Build history of the part. All positions in model axes, mm. A direction names the side the tool comes from. Coordinates: 2 decimals unless noted, no trailing zeros. Loops run counter-clockwise (first coordinate to the right, second up) from the corner with the lowest first, then second, coordinate; pieces in that order, holes last.
(1) Slice it at D-D (x = 38). Give the cut face in (y, z).
(2) Tool access for faces 4 (the face through (7, 13, 5)), 5 (the face through (-12.43, 14.15, 4.46)), 6 (the face through (35, 22, 5)), 7 (the face through (35, 3, 5)): list every direction of +Z, -Z, +X, -X, +Y, -Y with a clear straight run to the whole face (end or side of a thin tool).
(3) Flat gauge pins, fed straight in: P1, Ø3, axis at x = -6, y = 7, coming from the -Z side; P2, Ø4, axis at x = -3, y = 17.5, coming from the +Z side; P3, Ø5, axis at x = -3.5, z = 5, coming from the -Y side; P4, Ø7.5, axis at x = 39.5, z = 7, coming from the +Y side. Where does each tip first touch, or does it go through?
(4) Wall check: L1, parallel to X at y = 11.25, z = 5; L2, parallel to Y at x = 13, z = 6.25; L3, parallel to Z at x = 19, y = 5.25. Give the ranges that are in metal, low to high.
(5) Slice it at C-C (z = 5.75). Give the number of separate pieces and of enclosed holes in the cut face, and give its area (3 significant figures).
(6) Slice it at A-A (x = 19). Give the cut face in (y, z), and give its area (3 significant figures).
(7) Two-plate mould, pull along X, no slides. Class faces 1 (the face through (20.57, 4.563, 0.723)), 2 (the face through (2, 15, 10)), 3 (the face through (-12.4, 19.82, 4.46)): pulls with the +X half, pulls with the -X half, needs draft (parallel to the pull), parting line crosses it, or undercut.
(8) Slice it at B-B (z = 11.5). Give the cut face in (x, y).
Autodesk Inventor part; units mm, degrees
ref_plane "YZ Plane" through (0, 0, 0) normal (1, 0, 0) x (0, 1, 0)
ref_plane "XZ Plane" through (0, 0, 0) normal (0, 1, 0) x (-1, 0, 0)
ref_plane "XY Plane" through (0, 0, 0) normal (0, 0, 1) x (1, 0, 0)
sketch "Sketch1" plane through (0, 0, 0) normal (0, 0, 1) x (1, 0, 0)
  line L0 (0, 0) -> (0, 25)
  line L1 (0, 25) -> (35, 25)
  line L2 (35, 25) -> (35, 18.75)
  line L3 (35, 18.75) -> (44.5, 18.75)
  line L4 (44.5, 18.75) -> (44.5, 6.25)
  line L5 (44.5, 6.25) -> (35, 6.25)
  line L6 (35, 6.25) -> (35, 0)
  line L7 (35, 0) -> (0, 0)
  point P0 (0, 12.5)
  point P1 (44.5, 12.5)
  dimension "d0" = 25
  dimension "d1" = 35
  dimension "d2" = 12.5
  dimension "d3" = 6.25
  dimension "d4" = 9.5
extrude "Extrusion1" add sketch "Sketch1" along normal blind 10
hole "Hole1" at (40.2, 6.25, 5) direction (0, 1, 0) diameter 3 end through all
chamfer "Chamfer1" distance 2.5 angle 45 1 edges at (44.5, 12.5, 0)
hole "Hole2" at (19, 0, 4.51) direction (0, 1, 0) diameter 8.2 end through all
sketch "Sketch2" plane through (0, 0, 10) normal (0, 0, 1) x (1, 0, 0)
  line L0 (0, 25) -> (35, 25)
  line L1 (35, 0) -> (0, 0)
  line L2 (23.1, 25) -> (23.1, 0)
  line L3 (14.9, 25) -> (14.9, 0)
  line L4 (9, 0) -> (29, 0)
  line L5 (29, 0) -> (29, 25)
  line L6 (29, 25) -> (9, 25)
  line L7 (9, 25) -> (9, 0)
  dimension "d28" = 20
  dimension "d29" = 6
extrude "Extrusion2" add sketch "Sketch2" along normal blind 3
chamfer "Chamfer2" distance 3 angle 45 2 edges at (29, 12.5, 13) (9, 12.5, 13)
sketch "Sketch3" plane through (0, 0, 0) normal (-1, 0, 0) x (0, 0, 1)
  line L0 (10, 0) -> (10, 25)
  line L1 (0, 25) -> (10, 25)
  line L2 (10, 25) -> (10, 9)
  line L3 (10, 9) -> (0, 9)
  line L4 (0, 9) -> (0, 25)
  dimension "d35" = 16
extrude "Extrusion3" add sketch "Sketch3" along normal blind 13
hole "Hole3" at (-5.5, 17, 10) direction (0, 0, -1) diameter 4.5 end through all
sketch "Sketch4" plane through (0, 0, 10) normal (0, 0, 1) x (1, 0, 0)
  circle A0 centre (-5.5, 17) radius 2.25
  line L0 (-13, 25) -> (-13, 9)
  line L1 (-5.5, 19.25) -> (-13, 19.25)
  line L2 (-13, 19.25) -> (-13, 14.75)
  line L3 (-13, 14.75) -> (-5.5, 14.75)
  line L4 (-5.5, 14.75) -> (-5.5, 19.25)
extrude "Extrusion4" cut sketch "Sketch4" against normal through all contours L4 A0 | A0 L3 L0 L1 picked at (-6.2445, 17.0904)
fillet "Fillet1" radius 2 4 edges at (-13, 25, 5) (-13, 19.25, 5) (-13, 14.75, 5) (-13, 9, 5)
sketch "Sketch5" plane through (0, 9, 0) normal (0, -1, 0) x (1, 0, 0)
  line L0 (0, 10) -> (-11, 10)
  line L1 (-13, 10) -> (-13, 0)
  line L2 (-13, 10) -> (-11, 10)
  line L3 (-13, 10) -> (-9.4444, 10)
  line L4 (-13, 7.7985) -> (-13, 10)
  line L5 (-13, 7.7985) -> (-9.4444, 10)
  dimension "d52" = 3.5556
  dimension "d53" = 2.2015
extrude "Extrusion5" cut sketch "Sketch5" against normal through all
fillet "Fillet2" radius 6 1 edges at (0, 0, 5)
sketch "Sketch6" plane through (0, 0, 13) normal (0, 0, 1) x (1, 0, 0)
  line L0 (9, 0) -> (9, 25)
  line L1 (-9.4444, 25) -> (9, 25)
  line L2 (12, 25) -> (9, 25)
  line L3 (29, 25) -> (26, 25)
  line L4 (29, 25) -> (35, 25)
  line L5 (9, 0) -> (6, 0)
  line L6 (26, 0) -> (29, 0)
  line L7 (35, 0) -> (29, 0)
  line L8 (23.1, 25) -> (23.1, 0)
  line L9 (14.9, 25) -> (14.9, 0)
  line L10 (7, 9) -> (31, 9)
  line L11 (31, 9) -> (31, 17)
  line L12 (31, 17) -> (7, 17)
  line L13 (7, 17) -> (7, 9)
  point P0 (0, 0)
  dimension "d55" = 24
  dimension "d56" = 8
  dimension "d57" = 9
  dimension "d58" = 7.9
extrude "Extrusion6" cut sketch "Sketch6" against normal through all
chamfer "Chamfer3" distance 2 distance2 4 1 edges at (44.5, 12.5, 10) measured on face at (44.5, 14.5833, 5)
properties part number "idler mount"
Response values:
1. outline: (6.25, 0) - (18.75, 0) - (18.75, 10) - (6.25, 10) - close
2. face 4: +Z, -Z
2. face 5: +Z, -Z, -X
2. face 6: +Z, -Z, +X, +Y
2. face 7: +Z, -Z, +X, -Y
3. P1: passes through
3. P2: stops at z = 10
3. P3: stops at y = 9
3. P4: stops at y = 18.75
4. L1: x = -13 to 7, 31 to 38.7, 41.7 to 44.5
4. L2: y = 0 to 9, 17 to 25
4. L3: z = 0 to 0.41, 8.61 to 13
5. separate pieces: 3
5. enclosed holes: 0
5. area: 792 mm2
6. outline: (0, 0) - (9, 0) - (9, 0.41) - (0, 0.41) - close; (0, 8.61) - (9, 8.61) - (9, 13) - (0, 13) - close; (17, 0) - (25, 0) - (25, 0.41) - (17, 0.41) - close; (17, 8.61) - (25, 8.61) - (25, 13) - (17, 13) - close
6. area: 81.6 mm2
7. face 1: undercut
7. face 2: needs draft
7. face 3: pulls with the -X half
8. outline: (10.5, 0) - (27.5, 0) - (27.5, 9) - (10.5, 9) - close; (10.5, 17) - (27.5, 17) - (27.5, 25) - (10.5, 25) - close
